Verification items for the finished model (mm, model axes). Face numbers are marked on the shaded views. A direction names the side the tool comes from. Give positions to 0.01 mm unless a question says otherwise; leave off trailing zeros. Write each loop counter-clockwise with the first axis right and the second up, starting at its lowest first coordinate (ties: lowest second). Pieces come first, ordered by that corner, then holes. Notation, with made-up numbers: (-16, -24.5) -> (38, -24.5) arc R16 cw to (38, 6.5) -> close; hole circle Ø2 at (83.5, 10.25). An arc over 180 degrees is marked (long way). Use one line per item in the form item = value. Start each with the question number.
(1) Section check A-A, the plane z = 11. Record the cut outline in (x, y).
(2) Scan lines: L1, parallel to X at y = 0, z = 22.5; L2, parallel to Y at x = -34, z = 4.5; L3, parallel to Y at x = 34, z = 23.5. Record each from-to range of solid material in increasing order.
(3) Set-up check for the marked faces 5, 6 and 7: record each of +Z, -Z, +X, -X, +Y, -Y from which the full face is reachable in a straight line by a thin tool's end or side.
(4) Section check C-C, the plane x = -5.5. Record the cut outline in (y, z).
(5) Release check for a two-part mould opening along X. For the marked faces 1, 2, 3 and 4 record: pulls with the +X half, pulls with the -X half, needs draft (parallel to the pull), parting line crosses it, or undercut.
(6) Depth check by flat-ended pin: pin 1 Ø5 at (y, z) = (-3.5, 10.5) entering from -X (3 decimals); pin 2 Ø1 at (x, y) = (25.5, 32.5) entering from +Z; pin 3 Ø1 at (y, z) = (-11, 16.5) entering from +X; pin 4 Ø12.5 at (x, y) = (-34, 0) entering from -Z. Enter the tip coordinate at first touch or a pass-through.
(7) Section check B-B, the plane y = -13.5. Record the cut outline in (x, z).
(8) Section check D-D, the plane y = 13. Record the cut outline in (x, z).
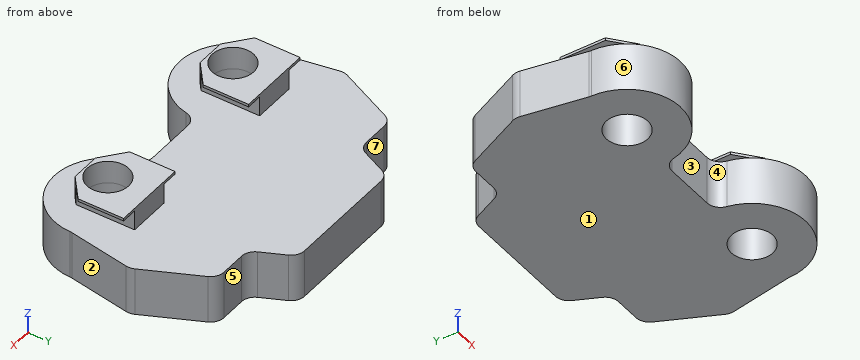
from build123d import *

# Parameters (mm, degrees)
CROQUIS1_R                 = 5.5
SALIENTE_EXTRUIR1_DEPTH    = 18
CORTAR_EXTRUIR1_DEPTH      = 89.71111533
CORTAR_EXTRUIR1_DEPTH_BACK = 89.71111533
CROQUIS2_R                 = 7.75
CROQUIS2_R_2               = 5.5
SALIENTE_EXTRUIR2_START    = 8.5
CROQUIS2_6_R               = 7.75
SALIENTE_EXTRUIR2_DEPTH    = 8.5
CROQUIS4_W                 = 7.5
CROQUIS4_H                 = 22.982035645
CORTAR_EXTRUIR2_DEPTH      = 6
CROQUIS5_W                 = 7.5
CROQUIS5_H                 = 22.982035645
CORTAR_EXTRUIR3_DEPTH      = 6


with BuildPart() as part:
    # Croquis1 → Saliente-Extruir1 (new body)
    with BuildSketch(Plane.XY):
        with BuildLine():
            Line((-9.505102572, 0), (9.505102572, 0))
            ThreePointArc((9.505102572, 0), (12.667380232, -1.127016654), (14.404082058, -4))
            ThreePointArc((14.404082058, -4), (35.826374721, -19.916434304), (53.996590294, -0.369292059))
            ThreePointArc((53.996590294, -0.369292059), (54.019000089, 0.020132875), (54.071699102, 0.406625814))
            Line((54.071699102, 0.406625814), (58.134419217, 23.447456541))
            ThreePointArc((58.134419217, 23.447456541), (58.167604759, 24.96832839), (57.741919387, 26.428788738))
            Line((57.741919387, 26.428788738), (48.108079819, 47.088624363))
            ThreePointArc((48.108079819, 47.088624363), (46.263038926, 49.192490284), (43.576540884, 49.975533055))
            Line((43.576540884, 49.975533055), (33.947243492, 49.975533055))
            ThreePointArc((33.947243492, 49.975533055), (31.26074545, 50.758575826), (29.415704557, 52.862441746))
            Line((29.415704557, 52.862441746), (25.346187631, 61.589548956))
            ThreePointArc((25.346187631, 61.589548956), (23.501146738, 63.693414876), (20.814648696, 64.476457647))
            Line((20.814648696, 64.476457647), (-20.814648696, 64.476457647))
            ThreePointArc((-20.814648696, 64.476457647), (-23.501146738, 63.693414876), (-25.346187631, 61.589548956))
            Line((-25.346187631, 61.589548956), (-29.415704557, 52.862441746))
            ThreePointArc((-29.415704557, 52.862441746), (-31.26074545, 50.758575826), (-33.947243492, 49.975533055))
            Line((-33.947243492, 49.975533055), (-43.576540884, 49.975533055))
            ThreePointArc((-43.576540884, 49.975533055), (-46.263038926, 49.192490284), (-48.108079819, 47.088624363))
            Line((-48.108079819, 47.088624363), (-57.741919387, 26.428788738))
            ThreePointArc((-57.741919387, 26.428788738), (-58.167604759, 24.96832839), (-58.134419217, 23.447456541))
            Line((-58.134419217, 23.447456541), (-54.071699102, 0.406625814))
            ThreePointArc((-54.071699102, 0.406625814), (-54.019000089, 0.020132875), (-53.996590294, -0.369292059))
            ThreePointArc((-53.996590294, -0.369292059), (-35.826374721, -19.916434304), (-14.404082058, -4))
            ThreePointArc((-14.404082058, -4), (-12.667380232, -1.127016654), (-9.505102572, 0))
        make_face()
        with Locations((34, 0)):
            Circle(CROQUIS1_R, mode=Mode.SUBTRACT)
        with Locations(Location((-34, 0, 0), (0, 0, 180))):
            Circle(CROQUIS1_R, mode=Mode.SUBTRACT)
    extrude(amount=SALIENTE_EXTRUIR1_DEPTH)

    # Croquis2 → Cortar-Extruir1 (cut, two sides: drawn at the far end of the back side and taken through both)
    # profile 1 of 2: a face of its own
    with BuildSketch(Plane.XY.offset(18).offset(-CORTAR_EXTRUIR1_DEPTH_BACK)):
        with Locations((-34, 0)):
            Circle(CROQUIS2_R)
        with Locations((-34, 0)):
            Circle(CROQUIS2_R_2, mode=Mode.SUBTRACT)
    # profile 2 of 2: a face of its own
    with BuildSketch(Plane.XY.offset(18).offset(-CORTAR_EXTRUIR1_DEPTH_BACK)):
        with Locations((34, 0)):
            Circle(CROQUIS2_R)
        with Locations((34, 0)):
            Circle(CROQUIS2_R_2, mode=Mode.SUBTRACT)
    extrude(amount=CORTAR_EXTRUIR1_DEPTH + CORTAR_EXTRUIR1_DEPTH_BACK, mode=Mode.SUBTRACT)

    # Croquis2_6 → Saliente-Extruir2 (add)
    # profile 1 of 2: a face of its own
    with BuildSketch(Plane.XY.offset(18).offset(SALIENTE_EXTRUIR2_START)):
        Polygon((-48.000069308, 15.502035645), (-19.999930692, 15.502035645), (-19.999930692, -1.497964355), (-28.5, -8.48), (-39.5, -8.48), (-48.000069308, -1.497964355), align=None)
        with Locations((-34, 0)):
            Circle(CROQUIS2_6_R, mode=Mode.SUBTRACT)
    # profile 2 of 2: a face of its own
    with BuildSketch(Plane.XY.offset(18).offset(SALIENTE_EXTRUIR2_START)):
        Polygon((19.999930692, -1.497964355), (19.999930692, 15.502035645), (48.000069308, 15.502035645), (48.000069308, -1.497964355), (39.5, -8.48), (28.5, -8.48), align=None)
        with Locations((34, 0)):
            Circle(CROQUIS2_6_R, mode=Mode.SUBTRACT)
    extrude(amount=-SALIENTE_EXTRUIR2_DEPTH)

    # Croquis4 → Cortar-Extruir2 (cut)
    with BuildSketch(Plane.ZY.offset(-19.999930692)):
        with Locations((21.75, 4.011017823)):
            Rectangle(CROQUIS4_W, CROQUIS4_H)
    cortar_extruir2 = extrude(amount=-CORTAR_EXTRUIR2_DEPTH, mode=Mode.SUBTRACT)

    # Croquis5 → Cortar-Extruir3 (cut)
    with BuildSketch(Plane(origin=(48.000069308, 0, 0), x_dir=(0, 0, -1), z_dir=(1, 0, 0))):
        with Locations((-21.75, 4.011017823)):
            Rectangle(CROQUIS5_W, CROQUIS5_H)
    cortar_extruir3 = extrude(amount=-CORTAR_EXTRUIR3_DEPTH, mode=Mode.SUBTRACT)

    # Simetr_a1: Cortar-Extruir2, Cortar-Extruir3 across plane
    add(cortar_extruir2.mirror(Plane(origin=(0, 0, 0), x_dir=(0, 0, 1), z_dir=(1, 0, 0))), mode=Mode.SUBTRACT)
    add(cortar_extruir3.mirror(Plane(origin=(0, 0, 0), x_dir=(0, 0, 1), z_dir=(1, 0, 0))), mode=Mode.SUBTRACT)


solid = part.part
Completed:
q1.outline = (-58.13, 23.45) -> (-54.07, 0.41) arc R5 cw to (-54, -0.37) arc R20 ccw to (-14.4, -4) arc R5 cw to (-9.51, 0) -> (9.51, 0) arc R5 cw to (14.4, -4) arc R20 ccw to (54, -0.37) arc R5 cw to (54.07, 0.41) -> (58.13, 23.45) arc R5 ccw to (57.74, 26.43) -> (48.11, 47.09) arc R5 ccw to (43.58, 49.98) -> (33.95, 49.98) arc R5 cw to (29.42, 52.86) -> (25.35, 61.59) arc R5 ccw to (20.81, 64.48) -> (-20.81, 64.48) arc R5 ccw to (-25.35, 61.59) -> (-29.42, 52.86) arc R5 cw to (-33.95, 49.98) -> (-43.58, 49.98) arc R5 ccw to (-48.11, 47.09) -> (-57.74, 26.43) arc R5 ccw to start; hole circle Ø15.5 at (-34, 0); hole circle Ø15.5 at (34, 0)
q2.L1 = -42 to -41.75, -26.25 to -26, 26 to 26.25, 41.75 to 42
q2.L2 = -20 to -7.75, 7.75 to 49.98
q2.L3 = -8.48 to -7.75, 7.75 to 15.5
q3.face_5 = +Z, -Z, +X, +Y
q3.face_6 = +Z, -Z, -Y
q3.face_7 = +Z, -Z, -X, +Y
q4.outline = (0, 0) -> (64.48, 0) -> (64.48, 18) -> (0, 18) -> close
q5.face_1 = needs draft
q5.face_2 = pulls with the +X half
q5.face_3 = undercut
q5.face_4 = undercut
q6.pin_1 = -53.975
q6.pin_2 = 18
q6.pin_3 = 51.02
q6.pin_4 = through
q7.outline = (-48.76, 0) -> (-19.24, 0) -> (-19.24, 18) -> (-48.76, 18) -> close; (19.24, 0) -> (48.76, 0) -> (48.76, 18) -> (19.24, 18) -> close
q8.outline = (-56.29, 0) -> (56.29, 0) -> (56.29, 18) -> (42, 18) -> (42, 25.5) -> (48, 25.5) -> (48, 26.5) -> (20, 26.5) -> (20, 25.5) -> (26, 25.5) -> (26, 18) -> (-26, 18) -> (-26, 25.5) -> (-20, 25.5) -> (-20, 26.5) -> (-48, 26.5) -> (-48, 25.5) -> (-42, 25.5) -> (-42, 18) -> (-56.29, 18) -> close
